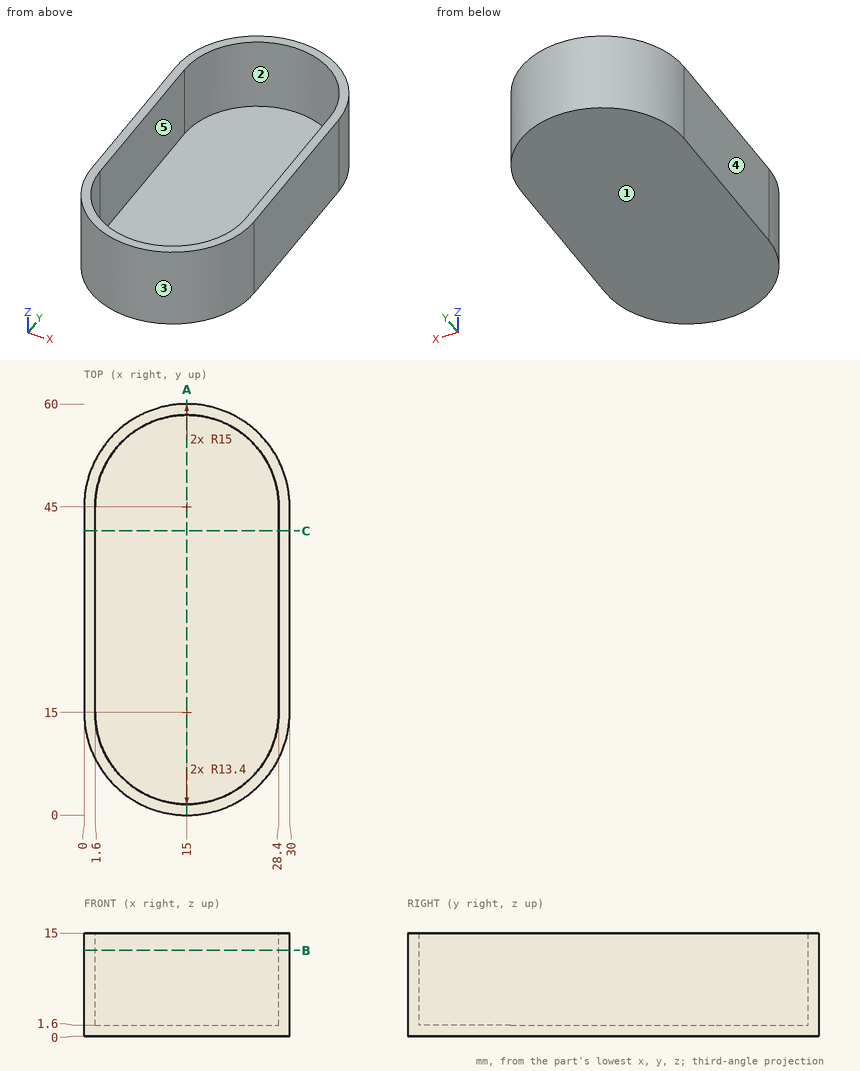
Design review of the part shown in the three views and the two pictorial views. Dimensions are in mm from the part's minimum x, y and z. A direction names the side the tool comes from. Round coordinates to 2 decimals unless told otherwise and drop trailing zeros. Write each loop counter-clockwise with the first axis right and the second up, starting at its lowest first coordinate (ties: lowest second). Pieces come first, ordered by that corner, then holes. Notation, with made-up numbers: (57.5, 32) - (92.5, 32) arc R25 cw to (92.5, 64) - close; hole circle Ø8 at (34.5, -20.5). An arc over 180 degrees is marked (long way). Write item = value, one per line. Start each with the question number.
1. Draft analysis for pull direction Y (two halves, no side actions). For the marked faces 1, 2 and 3, state which applies: released by +Y, released by -Y, zero draft, split by the parting line, or undercut.
2. Consider section A-A on x = 15. State the section outline as (y, z) points.
3. Consider section B-B on z = 12.5. State the section outline as (x, y) points, plus the area to 3 significant figures.
4. For pin 1 Ø10 at (x, y) = (12.5, 17) entering from -Z, flat-tipped, find the tip position at first contact; note if it passes through.
5. For the marked faces 4 and 5, list the 3-axis set-ups (+Z, -Z, +X, -X, +Y, -Y) from which the entire face can be reached by the end or side of a thin tool; tool diameter is ignored.
6. Wall thickness on L1, parallel to X at y = 38, z = 10.25; L2, parallel to Z at x = 15.75, y = 48; L3, parallel to Y at x = 24.5, z = 9: over which ranges is each line inside the solid? List them lowest first.
7. Consider section C-C on y = 41.5. State the section outline as (x, z) points, plus the area to 3 significant figures.
Evaluation:
q1.face_1 = zero draft
q1.face_2 = undercut
q1.face_3 = released by -Y
q2.outline = (0, 0) - (60, 0) - (60, 15) - (58.4, 15) - (58.4, 1.6) - (1.6, 1.6) - (1.6, 15) - (0, 15) - close
q3.outline = (0, 15) arc R15 ccw to (30, 15) - (30, 45) arc R15 ccw to (0, 45) - close; hole (1.6, 15) arc R13.4 ccw to (28.4, 15) - (28.4, 45) arc R13.4 ccw to (1.6, 45) - close
q3.area = 239 mm2
q4.pin_1 = 0
q5.face_4 = +Z, -Z, -X, +Y, -Y
q5.face_5 = +Z
q6.L1 = 0 to 1.6, 28.4 to 30
q6.L2 = 0 to 1.6
q6.L3 = 3.39 to 5.55, 54.45 to 56.61
q7.outline = (0, 0) - (30, 0) - (30, 15) - (28.4, 15) - (28.4, 1.6) - (1.6, 1.6) - (1.6, 15) - (0, 15) - close
q7.area = 90.9 mm2
